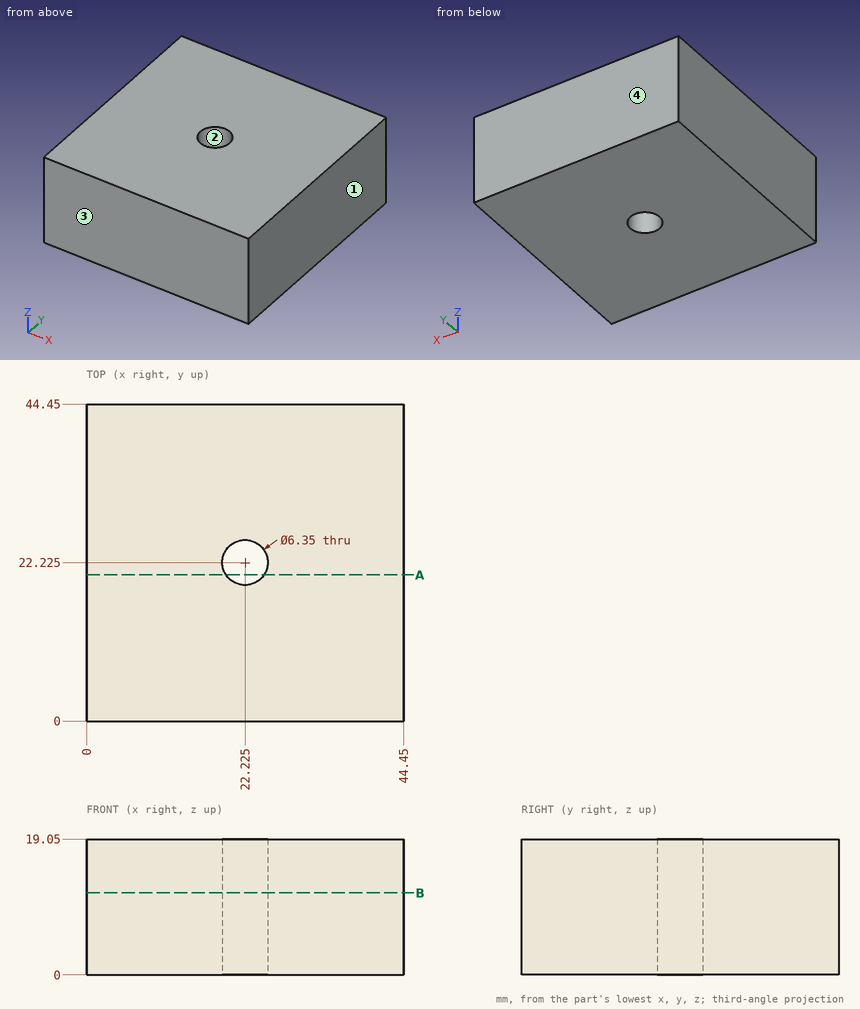
Can you work these out from the drawing? Everything is in mm from the part's minimum corner. Give positions to 0.01 mm unless a question says otherwise; leave off trailing zeros. Loops run counter-clockwise (first coordinate to the right, second up) from the corner with the lowest first, then second, coordinate; pieces in that order, holes last. Notation, with made-up numbers: (10, 14.5) -> (21, 14.5) arc R17 cw to (21, 37.5) -> close; hole circle Ø2 at (49, 69.5). An arc over 180 degrees is marked (long way). Return JSON: item names as keys, results as strings.
Item 1: If we section it at A-A on y = 20.5: List the corners of the cut face in (x, z) for me.
Geometry results:
{"outline": "(0, 0) -> (19.56, 0) -> (19.56, 19.05) -> (0, 19.05) -> close; (24.89, 0) -> (44.45, 0) -> (44.45, 19.05) -> (24.89, 19.05) -> close"}
Item 2: If we section it at B-B on z = 11.5: List the corners of the cut face in (x, y) for me (3 decimals).
Geometry results:
{"outline": "(0, 0) -> (44.45, 0) -> (44.45, 44.45) -> (0, 44.45) -> close; hole circle Ø6.35 at (22.225, 22.225)"}
Item 3: I'm going to push a flat-ended pin straight in: pin 1 (2 mm diameter, centred on y = 33.5, z = 8, fed in from -X). Where does the tip first touch, or does it pass through?
Geometry results:
{"pin 1": "stops at x = 0"}
Item 4: We'd pull the mould along Y, two halves only. Please class the marked faces 1, 2, 3 and 4: +Y half, -Y half, draft (parallel to the pull), parting line (faces both ways), or undercut.
Geometry results:
{"face 1": "draft", "face 2": "undercut", "face 3": "-Y half", "face 4": "+Y half"}
Item 5: I need wall thicknesses on L1, parallel to X at y = 19.5, z = 10.25; L2, parallel to X at y = 25, z = 1.25. Which ranges of each line are inside material? Lowest first, please. Write a range as from..to.
Geometry results:
{"L1": "x = 0..20.6, 23.85..44.45", "L2": "x = 0..20.68, 23.77..44.45"}
